Input: part model. Units: mm. Frame: model coordinates. A direction names the side the tool comes from. Round coordinates to 2 decimals unless told otherwise and drop trailing zeros. Loops run counter-clockwise (first coordinate to the right, second up) from the corner with the lowest first, then second, coordinate; pieces in that order, holes last.
(1) Cut plane B-B, the plane z = 11.5. Output: boundary loops of the cut face in (x, y), and give its area (3 significant figures).
(2) Line query: line 1 (Z direction, x = 14, y = 42.5); line 2 (X direction, y = 44, z = -7); line 3 (Y direction, x = 41, z = -8). Output: solid intervals per line, ascending.
(3) First-contact query: pin 1 Ø1.5 at (x, y) = (-30.5, 12) entering from +Z; pin 2 Ø2 at (y, z) = (26.5, -11.5) entering from -X; pin 3 Ø1.5 at (y, z) = (6, -21.5) entering from +X. Flat tips, straight axial feed; report the tip coordinate or a pass-through.
(4) Cut plane C-C, the plane y = 33. Output: boundary loops of the cut face in (x, z).
(5) Draft query along Z for faces 4 (the face through (-29.7, 44, 15.5)), 5 (the face through (-14.4, 45, -15.4)), 6 (the face through (-1.2, 43, -17.1)). Return one class per face: released by +Z, released by -Z, zero draft, split by the parting line, or undercut.
(6) Cut plane D-D, the plane z = 0. Output: boundary loops of the cut face in (x, y), and give its area (3 significant figures).
(7) Cut plane A-A, the plane x = 0. Output: boundary loops of the cut face in (y, z).
(8) Access query for faces 1 (the face through (-34.872, 40.535, 26.477)), 2 (the face through (14.718, 21.199, 46.737)), 3 (the face through (-13, 5, 40)). Directions: +Z, -Z, +X, -X, +Y, -Y. A direction counts if a zero-diameter tool reaches every point of the face in a straight line with its end or side. Return the directions, or none.
from build123d import *

# Parameters (mm, degrees)
SKETCH_1_R               = 49
EXTRUDE_1_DEPTH          = 43
SKETCH_2_R               = 33.5
EXTRUDE_2_DEPTH          = 2
SKETCH_4_R               = 20.5
EXTRUDE_4_DEPTH          = 0.5
SKETCH_5_R               = 2
CUT_EXTRUDE_1_DEPTH      = 5
PATTERN_CIRCULAR_1_COUNT = 6
SKETCH_6_R               = 2
CUT_EXTRUDE_2_DEPTH      = 5
PATTERN_CIRCULAR_2_COUNT = 10
CUT_EXTRUDE_START        = -5
SKETCH_7_R               = 2
CUT_EXTRUDE_3_DEPTH      = 5
PATTERN_CIRCULAR_3_COUNT = 10


with BuildPart() as part:
    # 草圖1 → 填料-伸長1 (new body)
    with BuildSketch(Plane(origin=(0, 0, 0), x_dir=(1, 0, 0), z_dir=(0, 1, 0))):
        with Locations(Location((0, 0, 0), (0, 0, 270))):
            Circle(SKETCH_1_R)
    extrude(amount=EXTRUDE_1_DEPTH)

    # 草圖2 → 填料-伸長2 (add)
    with BuildSketch(Plane(origin=(0, 43, 0), x_dir=(1, 0, 0), z_dir=(0, 1, 0))):
        with Locations(Location((0, 0, 0), (0, 0, 270))):
            Circle(SKETCH_2_R)
    extrude(amount=EXTRUDE_2_DEPTH)

    # 草圖4 → 填料-伸長4 (add)
    with BuildSketch(Plane(origin=(0, 45, 0), x_dir=(1, 0, 0), z_dir=(0, 1, 0))):
        with Locations(Location((0, 0, 0), (0, 0, 270))):
            Circle(SKETCH_4_R)
    extrude(amount=EXTRUDE_4_DEPTH)

    # 草圖5 → 除料-伸長1 (cut)
    with BuildSketch(Plane(origin=(0, 45.5, 0), x_dir=(1, 0, 0), z_dir=(0, 1, 0))):
        with Locations(Location((0, 15.5, 0), (0, 0, 270))):
            Circle(SKETCH_5_R)
    cut_extrude_1 = extrude(amount=-CUT_EXTRUDE_1_DEPTH, mode=Mode.SUBTRACT)

    # 環狀複製排列1: 除料-伸長1 ×6 about axis
    pattern_circular_1_axis = Axis((0, 0, 0), (0, 1, 0))
    for i in range(1, PATTERN_CIRCULAR_1_COUNT):
        add(cut_extrude_1.rotate(pattern_circular_1_axis, i * 360 / PATTERN_CIRCULAR_1_COUNT), mode=Mode.SUBTRACT)

    # 草圖6 → 除料-伸長2 (cut)
    with BuildSketch(Plane(origin=(0, 43, 0), x_dir=(1, 0, 0), z_dir=(0, 1, 0))):
        with Locations(Location((-42, 0, 0), (0, 0, 270))):
            Circle(SKETCH_6_R)
    cut_extrude_2 = extrude(amount=-CUT_EXTRUDE_2_DEPTH, mode=Mode.SUBTRACT)

    # 環狀複製排列2: 除料-伸長2 ×10 about axis
    pattern_circular_2_axis = Axis((0, 0, 0), (0, 1, 0))
    for i in range(1, PATTERN_CIRCULAR_2_COUNT):
        add(cut_extrude_2.rotate(pattern_circular_2_axis, i * 360 / PATTERN_CIRCULAR_2_COUNT), mode=Mode.SUBTRACT)

    # 草圖7 → 除料-伸長3 (cut)
    with BuildSketch(Plane.XZ.offset(CUT_EXTRUDE_START)):
        with Locations(Location((42, 0, 0), (0, 0, 270))):
            Circle(SKETCH_7_R)
    cut_extrude_3 = extrude(amount=CUT_EXTRUDE_3_DEPTH, mode=Mode.SUBTRACT)

    # 環狀複製排列3: 除料-伸長3 ×10 about axis
    pattern_circular_3_axis = Axis((0, 0, 0), (0, 1, 0))
    for i in range(1, PATTERN_CIRCULAR_3_COUNT):
        add(cut_extrude_3.rotate(pattern_circular_3_axis, i * 360 / PATTERN_CIRCULAR_3_COUNT), mode=Mode.SUBTRACT)


solid = part.part
Reported:
1. outline: (-47.63, 0) - (47.63, 0) - (47.63, 43) - (31.46, 43) - (31.46, 45) - (16.97, 45) - (16.97, 45.5) - (-16.97, 45.5) - (-16.97, 45) - (-31.46, 45) - (-31.46, 43) - (-47.63, 43) - close
1. area: 4,240 mm2
2. line 1: z = -46.96 to -41.66, -38.22 to -9.67, -5.83 to 5.83, 9.67 to 38.22, 41.66 to 46.96
2. line 2: x = -32.76 to -15.28, -11.57 to 11.57, 15.28 to 32.76
2. line 3: y = 0 to 43
3. pin 1: stops at z = 38.94
3. pin 2: stops at x = -47.86
3. pin 3: stops at x = 44.39
4. outline: circle Ø98 at (0, 0)
5. face 4: split by the parting line
5. face 5: zero draft
5. face 6: undercut
6. outline: (-49, 0) - (-44, 0) - (-44, 5) - (-40, 5) - (-40, 0) - (40, 0) - (40, 5) - (44, 5) - (44, 0) - (49, 0) - (49, 43) - (44, 43) - (44, 38) - (40, 38) - (40, 43) - (33.5, 43) - (33.5, 45) - (20.5, 45) - (20.5, 45.5) - (-20.5, 45.5) - (-20.5, 45) - (-33.5, 45) - (-33.5, 43) - (-40, 43) - (-40, 38) - (-44, 38) - (-44, 43) - (-49, 43) - close
6. area: 4,290 mm2
7. outline: (0, -49) - (43, -49) - (43, -33.5) - (45, -33.5) - (45, -20.5) - (45.5, -20.5) - (45.5, -17.5) - (40.5, -17.5) - (40.5, -13.5) - (45.5, -13.5) - (45.5, 13.5) - (40.5, 13.5) - (40.5, 17.5) - (45.5, 17.5) - (45.5, 20.5) - (45, 20.5) - (45, 33.5) - (43, 33.5) - (43, 49) - (0, 49) - close
8. face 1: +Y
8. face 2: +Y, -Y
8. face 3: -Y
